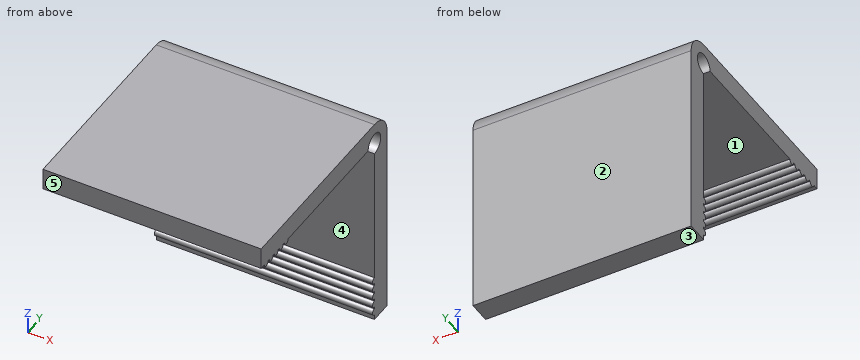
Autodesk Fusion 360 part; units mm, degrees
sketch "Sketch1" plane through (0, 0, 0) normal (1, 0, 0) x (0, 1, 0)
  line L0 (0, 0) -> (-166.0515, 0)
  line L1 (-166.0515, 0) -> (-166.0515, -106.0261)
  line L2 (-166.0515, -106.0261) -> (0, -106.0261)
  line L3 (0, -106.0261) -> (0, 0)
  line L4 (-90, 0) -> (-90, 10)
  line L5 (-90, 10) -> (0, 10)
  line L6 (10, 0) -> (10, -90)
  line L7 (10, -90) -> (0, -90)
  circle A0 centre (0, 0) radius 5
  arc A1 (10, 0) -> (0, 10) centre (0, 0) ccw
  circle A2 centre (-70, 0) radius 1.5
  circle A3 centre (-74, 0) radius 1.5
  circle A4 centre (-78, 0) radius 1.5
  circle A5 centre (-82, 0) radius 1.5
  circle A6 centre (-86, 0) radius 1.5
  line L8 (-86, 0) -> (-82, 0)
  line L9 (-86, 0) -> (-90, 0)
  line L10 (-82, 0) -> (-78, 0)
  line L11 (-78, 0) -> (-74, 0)
  line L12 (-74, 0) -> (-70, 0)
  line L13 (0, 0) -> (7.0711, 7.0711)
  circle A7 centre (0, -86) radius 1.5
  circle A8 centre (0, -82) radius 1.5
  circle A9 centre (0, -78) radius 1.5
  circle A10 centre (0, -74) radius 1.5
  circle A11 centre (0, -70) radius 1.5
  point P0 (10, 10)
  point P1 (-65.366, 0)
  dimension "d1" = 10
  dimension "d2" = 100
  dimension "d5" = 10
  dimension "d6" = 10
  dimension "d7" = 3
  dimension "d8" = 4
extrude "Extrude1" add sketch "Sketch1" along normal blind 100 contours L0 A2 L12 | L0 L4 L5 A0 A1 A2 A3 A4 A5 A6 L8 L9 L10 L11 L12 L13 | L0 A2 L12 | L3 L6 L7 A0 A1 L13 A7 A8 A9 A10 A11 | L0 A3 L11 L12 | L0 A3 L11 L12 | L3 A11 | L3 A11 | L0 A4 L10 L11 | L0 A4 L10 L11 | L3 A10 | L3 A10 | L0 A5 L8 L10 | L0 A5 L8 L10 | L3 A7 | L3 A7 | L0 A6 L8 L9 | L0 A6 L8 L9 | L3 A9 | L3 A9 | L3 A8 | L3 A8
The model under review builds one solid part; all positions refer to its coordinate system, in mm. Face numbers are marked on the shaded views. A direction names the side the tool comes from. Round coordinates to 2 decimals unless told otherwise and drop trailing zeros. Loops run counter-clockwise (first coordinate to the right, second up) from the corner with the lowest first, then second, coordinate; pieces in that order, holes last. Notation, with made-up numbers: M -25.75,-3.75 L -21.75,-3.75 A19 ccw -21.75,10.25 Z; hole C 39,18.25 d6. An arc over 180 degrees is marked long. Answer as CSV lines item,"result". Start each with the question number.
Item 1: Wall thickness on line 1 (Z direction, x = 29.5, y = -0.5); line 2 (Z direction, x = 15.5, y = -42); line 3 (Y direction, x = 95, z = -70): over which ranges is each line inside the solid? List them lowest first. Write a range as [from, to].
Item 2: Consider section B-B (y = -10.5). Write out the cut boundary in (x, z), then the cut area to 3 significant figures.
Item 3: For the marked faces 4 and 5, list the 3-axis set-ups (+Z, -Z, +X, -X, +Y, -Y) from which the entire face can be reached by the end or side of a thin tool; tool diameter is ignored.
Item 4: Mouldability with a two-part tool opening along Y and no side actions: class the marked faces 1, 2 and 3 as released by +Y, released by -Y, zero draft, split by the parting line, or undercut.
Item 5: Insertion check: P1, Ø2, axis at x = 52, z = -89, coming from the -Y side; P2, Ø4, axis at x = 77.5, y = -9, coming from the -Z side; P3, Ø9, axis at y = 0, z = 0, coming from the -X side; P4, Ø5, axis at x = 75.5, y = -76, coming from the -Z side. Each pin has a flat end and moves straight along its axis. Give the tip position at first contact, or say it passes through.
Item 6: Consider section A-A (x = 40). Write out the cut boundary in (y, z).
Answer:
1,line 1,"z = [-87.41, -84.59], [-83.41, -80.59], [-79.41, -76.59], [-75.41, -72.59], [-71.41, -68.59], [4.97, 10]"
1,line 2,"z = [0, 10]"
1,line 3,"y = [-1.5, 10]"
2,outline,"M 0,0 L 100,0 L 100,10 L 0,10 Z"
2,area,"1,000 mm^2"
3,face 4,"+X, -X, -Y"
3,face 5,"+Z, -Z, +X, -X, -Y"
4,face 1,"undercut"
4,face 2,"released by +Y"
4,face 3,"zero draft"
5,P1,"stops at y = 0"
5,P2,"stops at z = 0"
5,P3,"passes through"
5,P4,"stops at z = -1.5"
6,outline,"M -90,0 L -87.5,0 A1.5 ccw -84.5,0 L -83.5,0 A1.5 ccw -80.5,0 L -79.5,0 A1.5 ccw -76.5,0 L -75.5,0 A1.5 ccw -72.5,0 L -71.5,0 A1.5 ccw -68.5,0 L -5,0 A5 cw long 0,-5 L 0,-68.5 A1.5 ccw 0,-71.5 L 0,-72.5 A1.5 ccw 0,-75.5 L 0,-76.5 A1.5 ccw 0,-79.5 L 0,-80.5 A1.5 ccw 0,-83.5 L 0,-84.5 A1.5 ccw 0,-87.5 L 0,-90 L 10,-90 L 10,0 A10 ccw 0,10 L -90,10 Z"
